from build123d import *

# Parameters (mm, degrees)
SKETCH1_R               = 40
BOSS_EXTRUDE1_DEPTH     = 30
FILLET1_R               = 10
CUT_EXTRUDE1_DEPTH      = 65.031242437
CUT_EXTRUDE1_DEPTH_BACK = 65.031242437
SKETCH2_R               = 5


with BuildPart() as part:
    # Sketch1 → Boss-Extrude1 (new body)
    with BuildSketch(Plane.XY):
        Circle(SKETCH1_R)
    extrude(amount=BOSS_EXTRUDE1_DEPTH)

    # Fillet1
    fillet1_edges = [part.edges().sort_by_distance(p)[0] for p in [
        (-40, 0, 0),
        (-40, 0, 30),
    ]]
    fillet(fillet1_edges, radius=FILLET1_R)

    # Sketch2 → Cut-Extrude1 (cut, two sides: drawn at the far end of the back side and taken through both)
    with BuildSketch(Plane.XY.offset(30).offset(-CUT_EXTRUDE1_DEPTH_BACK)):
        Circle(SKETCH2_R)
    extrude(amount=CUT_EXTRUDE1_DEPTH + CUT_EXTRUDE1_DEPTH_BACK, mode=Mode.SUBTRACT)


solid = part.part
Verification items for the finished model (mm, model axes). Coordinates: 2 decimals unless noted, no trailing zeros. Order: outer loops, then holes, each group sorted by start corner. A loop starts at its lowest first (then second) coordinate and runs counter-clockwise, first axis right, second up. Notation, with made-up numbers: M -31.5,-22.5 L 7.5,-22.5 A31 cw 7.5,9.5 Z; hole C 46,-15 d11. An arc over 180 degrees is marked long. Write each question's results on one line, items separated by ' | '.
1) Scan lines: line 1 along Y through (x, z) = (0, 12.75); line 2 along X through (y, z) = (-0.5, 17); line 3 along Y through (x, z) = (0, 22). Record each from-to range of solid material in increasing order. Write a range as [from, to].
Solved:
line 1: y = [-40, -5], [5, 40] | line 2: x = [-40, -4.97], [4.97, 40] | line 3: y = [-39.8, -5], [5, 39.8]
2) Section check C-C on z = 12. Record the cut outline in (x, y).
Solved:
outline: C 0,0 d80; hole C 0,0 d10
3) Gauge pin test, flat ends, axial feed: pin 1 Ø1.5 at (x, z) = (-23, 16.5) entering from -Y; pin 2 Ø16 at (x, y) = (0, 0) entering from -Z; pin 3 Ø3 at (y, z) = (-5.5, 14.5) entering from +X; pin 4 Ø4 at (x, z) = (-16.5, 7.5) entering from +Y. Record the tip position at first contact, or that the pin passes through.
Solved:
pin 1: stops at y = -33.24 | pin 2: stops at z = 0 | pin 3: stops at x = 39.8 | pin 4: stops at y = 37.06
4) Release check for a two-part mould opening along X. For faces 1 (the face through (0, -6, 30)), 2 (the face through (-1.08, -4.88, 14.79)), 3 (the face through (-8.67, -39.05, 14.93)) record: pulls with the +X half, pulls with the -X half, needs draft (parallel to the pull), parting line crosses it, or undercut.
Solved:
face 1: needs draft | face 2: undercut | face 3: parting line crosses it
5) Section check A-A on y = 0. Record the cut outline in (x, z), plus the area to 3 significant figures.
Solved:
outline: M -40,10 A10 ccw -30,0 L -5,0 L -5,30 L -30,30 A10 ccw -40,20 Z; M 5,0 L 30,0 A10 ccw 40,10 L 40,20 A10 ccw 30,30 L 5,30 Z | area: 2,010 mm²
